The listing builds one solid part. Answer for the finished solid, in the listing's coordinates (mm). Face numbers are marked on the shaded views. A direction names the side the tool comes from. Give positions to 0.01 mm unless a question says otherwise; leave off trailing zeros. Loops run counter-clockwise (first coordinate to the right, second up) from the corner with the lowest first, then second, coordinate; pieces in that order, holes last. Notation, with made-up numbers: M -6.75,-20 L 35.25,-20 A4 ccw 35.25,-14 Z; hole C -20.5,8.5 d6. An arc over 180 degrees is marked long. Use one line per item in the form item = value. Start each with the question number.
1. The part is cut by section B-B (y = -24). Give the number of separate pieces and of enclosed holes in the cut face, and give its area (3 significant figures).
2. The part is cut by section C-C (x = -7.75). Write down the section's boundary in (y, z), and give its area (3 significant figures).
3. For the marked faces 1, 2 and 3, determine the directions among +Z, -Z, +X, -X, +Y, -Y from which every point of the face is accessible in a straight line to the end or side of a thin tool.
4. Straight lines are drawn through the part: line 1 (X direction, y = -24, z = -3.1); line 2 (X direction, y = -8, z = -2.4); line 3 (Y direction, x = -8, z = 2.7). For each, find the intervals that lie inside material, in ascending order. Write a range as from..to.
5. The mould has two halves that part along X. Classify the marked faces 4, 5 and 6: released by +X, released by -X, zero draft, split by the parting line, or undercut.
6. The part is cut by section A-A (x = -4). Write down the section's boundary in (y, z).
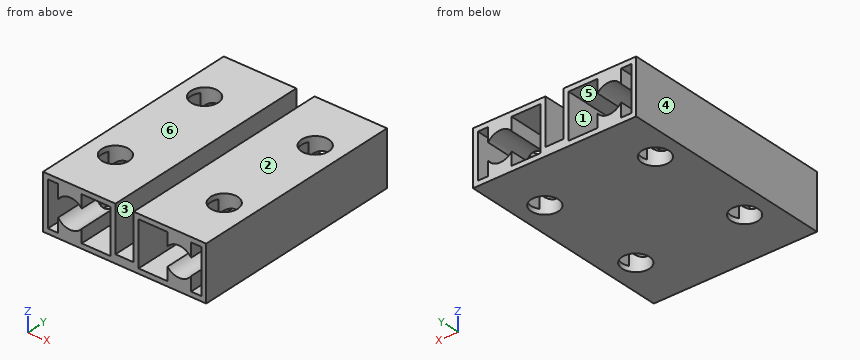
from build123d import *

# Parameters (mm, degrees)
F1_DEPTH = 32
F2_R     = 2
F3_DEPTH = 8.1


with BuildPart() as f1:
    # F0 (on Front) → F1 (new body)
    with BuildSketch(Plane.XZ):
        Polygon((-1.34, 4), (-12, 4), (-12, -4), (12, -4), (12, 4), (1.34, 4), (1.34, -2.75), (-1.34, -2.75), align=None)
        Polygon((-6.31, 3.28), (-2.06, 3.28), (-2.06, -3.28), (-6.31, -3.28), (-9.78, -3.28), (-11.28, -3.28), (-11.28, 3.28), (-9.78, 3.28), align=None, mode=Mode.SUBTRACT)
        Polygon((11.28, 3.28), (11.28, -3.28), (9.78, -3.28), (6.31, -3.28), (2.06, -3.28), (2.06, 3.28), (6.31, 3.28), (9.78, 3.28), align=None, mode=Mode.SUBTRACT)
        with BuildLine():
            Line((-6.31, 1.345177), (-6.31, 3.28))
            Line((-6.31, 3.28), (-9.78, 3.28))
            Line((-9.78, 3.28), (-9.78, 1.223601))
            ThreePointArc((-9.78, 1.223601), (-8.075632, 2.158675), (-6.31, 1.345177))
        make_face()
        with BuildLine():
            Line((-9.78, -3.28), (-6.31, -3.28))
            Line((-6.31, -3.28), (-6.31, -1.345177))
            ThreePointArc((-6.31, -1.345177), (-8.075632, -2.158675), (-9.78, -1.223601))
            Line((-9.78, -1.223601), (-9.78, -3.28))
        make_face()
        with BuildLine():
            Line((9.78, 1.223601), (9.78, 3.28))
            Line((9.78, 3.28), (6.31, 3.28))
            Line((6.31, 3.28), (6.31, 1.345177))
            ThreePointArc((6.31, 1.345177), (8.075632, 2.158675), (9.78, 1.223601))
        make_face()
        with BuildLine():
            Line((6.31, -3.28), (9.78, -3.28))
            Line((9.78, -3.28), (9.78, -1.223601))
            ThreePointArc((9.78, -1.223601), (8.075632, -2.158675), (6.31, -1.345177))
            Line((6.31, -1.345177), (6.31, -3.28))
        make_face()
    extrude(amount=F1_DEPTH)

    # F2 (on face) → F3 (cut)
    with BuildSketch(Plane.XY.offset(4)):
        with Locations((-8, -24)):
            Circle(F2_R)
        with Locations((8, -24)):
            Circle(F2_R)
        with Locations((-8.176223, -8)):
            Circle(F2_R)
        with Locations((8.085492, -8)):
            Circle(F2_R)
    extrude(amount=-F3_DEPTH, mode=Mode.SUBTRACT)


solid = f1.part
Derived:
q1.separate_pieces = 3
q1.enclosed_holes = 0
q1.area = 41.4 mm2
q2.outline = M -32,-4 L -25.98,-4 L -25.98,-2.15 L -32,-2.15 Z; M -32,2.15 L -25.98,2.15 L -25.98,4 L -32,4 Z; M -22.02,-4 L -9.95,-4 L -9.95,-2.15 L -22.02,-2.15 Z; M -22.02,2.15 L -9.95,2.15 L -9.95,4 L -22.02,4 Z; M -6.05,-4 L 0,-4 L 0,-2.15 L -6.05,-2.15 Z; M -6.05,2.15 L 0,2.15 L 0,4 L -6.05,4 Z
q2.area = 89.5 mm2
q3.face_1 = +Y, -Y
q3.face_2 = +Z, +X, -X, +Y, -Y
q3.face_3 = +Z, +Y, -Y
q4.line_1 = -12..-11.28, -2.06..2.06, 11.28..12
q4.line_2 = -12..-11.28, -2.06..-1.34, 1.34..2.06, 11.28..12
q4.line_3 = -32..-26, -22..-9.99, -6.01..0
q5.face_4 = released by -X
q5.face_5 = undercut
q5.face_6 = zero draft
q6.outline = M -32,-4 L 0,-4 L 0,-3.28 L -32,-3.28 Z; M -32,3.28 L 0,3.28 L 0,4 L -32,4 Z
